Can you work these out from the model? Positions are in its coordinate system, mm. A direction names the side the tool comes from. Give positions to 0.01 mm unless a question says otherwise; leave off trailing zeros. Loops run counter-clockwise (first coordinate to the right, second up) from the corner with the lowest first, then second, coordinate; pieces in that order, holes last. Notation, with made-up numbers: (24.25, 16.5) - (81.25, 16.5) arc R23 ccw to (81.25, 50.5) - close; hole circle Ø10 at (-24.75, 68.25). An arc over 180 degrees is marked (long way). Answer as a JSON object with one key per item and string values.
```python
from build123d import *

# Parameters (mm, degrees)
SKETCH1_R           = 3.175
BOSS_EXTRUDE1_DEPTH = 4.7752
FILLET1_R           = 3.175
SKETCH2_R           = 1.5875
CUT_EXTRUDE2_DEPTH  = 12.6492


with BuildPart() as part:
    # Sketch1 → Boss-Extrude1 (new body)
    with BuildSketch(Plane.XY):
        with BuildLine():
            ThreePointArc((-41.708677179, -11.175806368), (-39.414754754, -14.217464212), (-35.65126732, -14.809008693))
            Line((-35.65126732, -14.809008693), (-16.055699309, -10.252659153))
            ThreePointArc((-16.055699309, -10.252659153), (8.35578547, -17.119677251), (17.960512242, 6.35))
            Line((17.960512242, 6.35), (50.8, 6.35))
            ThreePointArc((50.8, 6.35), (80.4348452, 18.6251548), (92.71, 48.26))
            Line((92.71, 48.26), (92.71, 83.82))
            Line((92.71, 83.82), (80.01, 83.82))
            Line((80.01, 83.82), (48.380818336, 86.587194832))
            Line((48.380818336, 86.587194832), (47.273940403, 73.935522166))
            Line((47.273940403, 73.935522166), (80.01, 71.071488063))
            Line((80.01, 71.071488063), (80.01, 48.26))
            ThreePointArc((80.01, 48.26), (71.454589078, 27.605410922), (50.8, 19.05))
            Line((50.8, 19.05), (0, 19.05))
            ThreePointArc((0, 19.05), (-9.153942952, 16.706520536), (-16.055699309, 10.252659153))
            Line((-16.055699309, 10.252659153), (-35.65126732, 14.809008693))
            ThreePointArc((-35.65126732, 14.809008693), (-39.414754754, 14.217464212), (-41.708677179, 11.175806368))
            ThreePointArc((-41.708677179, 11.175806368), (-43.18, 0), (-41.708677179, -11.175806368))
        make_face()
        with BuildLine():
            ThreePointArc((-23.921153088, -6.409653652), (-26.166217118, -10.298218619), (-30.054782085, -8.053154588))
            ThreePointArc((-30.054782085, -8.053154588), (-31.115, 0), (-30.054782085, 8.053154588))
            ThreePointArc((-30.054782085, 8.053154588), (-26.166217118, 10.298218619), (-23.921153088, 6.409653652))
            ThreePointArc((-23.921153088, 6.409653652), (-24.765, 0), (-23.921153088, -6.409653652))
        make_face(mode=Mode.SUBTRACT)
        with BuildLine():
            ThreePointArc((-20.24097569, -5.42355309), (-20.955, 0), (-20.24097569, 5.42355309))
            ThreePointArc((-20.24097569, 5.42355309), (-16.352410723, 7.66861712), (-14.107346693, 3.780052154))
            ThreePointArc((-14.107346693, 3.780052154), (-14.605, 0), (-14.107346693, -3.780052154))
            ThreePointArc((-14.107346693, -3.780052154), (-16.352410723, -7.66861712), (-20.24097569, -5.42355309))
        make_face(mode=Mode.SUBTRACT)
        with Locations((-38.1, 0)):
            Circle(SKETCH1_R, mode=Mode.SUBTRACT)
        with BuildLine():
            ThreePointArc((1.438133327, 6.185003843), (-0.723783669, -6.308616108), (0, 6.35))
            Line((0, 6.35), (0.728531617, 6.35))
            Line((0.728531617, 6.35), (1.438133327, 6.185003843))
        make_face(mode=Mode.SUBTRACT)
    extrude(amount=BOSS_EXTRUDE1_DEPTH)

    # Fillet1
    # the kernel refuses this fillet: 3.175 mm, written as the material it adds along each edge
    with BuildSketch(Plane(origin=(-16.055699309, 10.252659153, 0), x_dir=(0.5808999309278821, 0.8139749813403246, 0), z_dir=(0, 0, 1))) as fillet1_piece_1:
        with BuildLine():
            CenterArc((2.126250916, 3.170784423), FILLET1_R, 202.42407708, 64.623066475)
            Line((-0.808674052, 1.959652545), (0, 0))
            ThreePointArc((0, 0), (0.981346577, 0.025293461), (1.962693154, 0))
        make_face()
    extrude(amount=4.7752)
    with BuildSketch(Plane(origin=(80.01, 71.071488063, 0), x_dir=(-0.9961946980917454, 0.08715574274765892, 0), z_dir=(0, 0, 1))) as fillet1_piece_2:
        with BuildLine():
            CenterArc((FILLET1_R * 0.916331174017, FILLET1_R), FILLET1_R, 185, 85)
            Line((-FILLET1_R * 0.0798635240743, FILLET1_R * 0.912844257252), (0, 0))
            Line((0, 0), (FILLET1_R * 0.916331174017, 0))
        make_face()
    extrude(amount=4.7752)
    with BuildSketch(Plane(origin=(80.01, 83.82, 0), x_dir=(1, 0, 0), z_dir=(0, 0, 1))) as fillet1_piece_3:
        with BuildLine():
            CenterArc((FILLET1_R * 0.0436609429085, FILLET1_R), FILLET1_R, 265, 5)
            Line((-FILLET1_R * 0.0434947998391, FILLET1_R * 0.00380530190826), (0, 0))
            Line((0, 0), (FILLET1_R * 0.0436609429085, 0))
        make_face()
    extrude(amount=4.7752)
    with BuildSketch(Plane(origin=(17.960512242, 6.35, 0), x_dir=(0.23924892683917381, -0.9709582642968253, 0), z_dir=(0, 0, 1))) as fillet1_piece_4:
        with BuildLine():
            CenterArc((4.048528681, 3.159689746), FILLET1_R, 166.157784332, 98.213210702)
            Line((0.965736192, 3.919305089), (0, 0))
            ThreePointArc((0, 0), (1.868551699, 0.091861522), (3.737103398, 0))
        make_face()
    extrude(amount=4.7752)
    with BuildSketch(Plane(origin=(-16.055699309, -10.252659153, 0), x_dir=(-0.9740163531879217, -0.22647768923781808, 0), z_dir=(0, 0, 1))) as fillet1_piece_5:
        with BuildLine():
            CenterArc((2.1199509, 3.175), FILLET1_R, 205.376933525, 64.623066475)
            ThreePointArc((-0.748686692, 1.814285714), (-0.350962429, 0.916791272), (0, 0))
            Line((0, 0), (2.1199509, 0))
        make_face()
    extrude(amount=4.7752)
    # the kernel refuses this fillet: 3.175 mm, written as the material it takes off along each edge
    with BuildSketch(Plane(origin=(47.273940403, 73.935522166, -7.9375), x_dir=(0.0871557427476583, 0.9961946980917454, 0), z_dir=(0, 0, 1)), Plane(origin=(48.380818336, 86.587194832, -7.9375), x_dir=(0.9961946980917455, -0.08715574274765811, 0), z_dir=(0, 0, 1)), Plane(origin=(92.71, 83.82, -7.9375), x_dir=(0, -1, 0), z_dir=(0, 0, 1))) as fillet1_2_piece_1:
        with BuildLine():
            CenterArc((FILLET1_R, -FILLET1_R), FILLET1_R, 90, 90)
            Line((0, -FILLET1_R), (0, 0))
            Line((0, 0), (FILLET1_R, 0))
        make_face()
    extrude(amount=20.6502, mode=Mode.SUBTRACT)

    # Sketch2 → Cut-Extrude2 (cut)
    with BuildSketch(Plane.XY.offset(4.7752)):
        with Locations((0, 12.7)):
            Circle(SKETCH2_R)
        with Locations((0, -12.7)):
            Circle(SKETCH2_R)
        with Locations((25.4, 12.7)):
            Circle(SKETCH2_R)
        with Locations((54.153215702, 79.707919533)):
            Circle(SKETCH2_R)
        with Locations((50.8, 12.7)):
            Circle(SKETCH2_R)
        with Locations((86.36, 77.47)):
            Circle(SKETCH2_R)
        with Locations((86.36, 48.26)):
            Circle(SKETCH2_R)
    extrude(amount=-CUT_EXTRUDE2_DEPTH, mode=Mode.SUBTRACT)


solid = part.part
```
1) Imagine slicing it at D-D on y = 38. Write out the boundary of the cut face in (x, z).
Check sheet entries:
{"outline": "(78.15, 0) - (91.43, 0) - (91.43, 4.78) - (78.15, 4.78) - close"}
2) Imagine slicing it at B-B on x = 86.36. Write out the boundary of the cut face in (y, z).
Check sheet entries:
{"outline": "(26.08, 0) - (46.67, 0) - (46.67, 4.78) - (26.08, 4.78) - close; (49.85, 0) - (75.88, 0) - (75.88, 4.78) - (49.85, 4.78) - close; (79.06, 0) - (83.82, 0) - (83.82, 4.78) - (79.06, 4.78) - close"}
3) I need wall thicknesses on L1, parallel to Y at x = 0, z = 2.5; L2, parallel to X at y = -1, z = 2.75; L3, parallel to X at y = 77.47, z = 2.8. Which ranges of each line are inside material? Lowest first, please.
Check sheet entries:
{"L1": "-19.05 to -14.29, -11.11 to -6.35, 6.35 to 11.11, 14.29 to 19.05", "L2": "-43.17 to -41.11, -35.09 to -31.1, -24.74 to -20.93, -14.57 to -6.27, 6.27 to 19.02", "L3": "47.58 to 84.77, 87.95 to 92.71"}
4) Which directions (+Z, -Z, +X, -X, +Y, -Y) give clear straight access to the entire face, cutting with the end or side of a thin tool? Please do faces 4 (the cylindrical face through (79.2, 70.28, 2.35)), 5 (the cylindrical face through (-31.115, -0.114, 2.354)), 6 (the flat face through (35, 18, 0)).
Check sheet entries:
{"face 4": "+Z, -Z, -X", "face 5": "+Z, -Z", "face 6": "-Z, +X, -X, +Y, -Y"}
5) Imagine slicing it at C-C on x = -38.1. Write out the boundary of the cut face in (y, z) (3 decimals), and give its area (3 significant figures).
Check sheet entries:
{"outline": "(-14.772, 0) - (-3.175, 0) - (-3.175, 4.775) - (-14.772, 4.775) - close; (3.175, 0) - (14.772, 0) - (14.772, 4.775) - (3.175, 4.775) - close", "area": "111 mm2"}
6) If we mould it in two halves opening along Y, with no side actions, what happens to faces 1 (the cylindrical face through (87.826, 76.862, 2.421)), 2 (the cylindrical face through (80.107, 18.301, 2.354)), 3 (the cylindrical face through (-8.17, 17.21, 2.35))? For each: released by +Y, released by -Y, zero draft, split by the parting line, or undercut.
Check sheet entries:
{"face 1": "undercut", "face 2": "released by -Y", "face 3": "released by +Y"}
7) Imagine slicing it at A-A on x = 25.4. Write out the boundary of the cut face in (y, z).
Check sheet entries:
{"outline": "(6.35, 0) - (11.11, 0) - (11.11, 4.78) - (6.35, 4.78) - close; (14.29, 0) - (19.05, 0) - (19.05, 4.78) - (14.29, 4.78) - close"}
8) I'm going to push flat-ended pins straight in: P1, Ø1.5, axis at x = 42.5, z = 3, coming from the +Y side; P2, Ø1.5, axis at y = 38.5, z = 2, coming from the +X side; P3, Ø2.5, axis at x = 16.5, z = 3, coming from the +Y side. Where does each tip first touch, or does it pass through?
Check sheet entries:
{"P1": "y = 19.05", "P2": "x = 91.73", "P3": "y = 19.05"}
